```python
from build123d import *

# Parameters (mm, degrees)
SKETCH2_W             = 76.2
SKETCH2_H             = 6.15
BOSS_EXTRUDE1_DEPTH   = 28.575
BOSS_EXTRUDE1_2_DEPTH = 28.575
SKETCH2_3_W           = 76.2
SKETCH2_3_H           = 12.9
BOSS_EXTRUDE2_DEPTH   = 3.175
CUT_EXTRUDE2_DEPTH    = 90.858670283
SKETCH4_R             = 3.175
SKETCH4_R_2           = 2.38125
SKETCH4_R_3           = 1.5875
SKETCH4_R_4           = 0.79375
CUT_EXTRUDE3_DEPTH    = 90.858670283
SKETCH5_R             = 0.2
CUT_EXTRUDE4_DEPTH    = 90.858670283
CHAMFER1_SIZE         = 0.4
SKETCH6_W             = 76.2
SKETCH6_H             = 1
CUT_EXTRUDE5_DEPTH    = 0.79375


with BuildPart() as part:
    # Sketch2 → Boss-Extrude1 (new body)
    with BuildSketch(Plane(origin=(0, 0, 0), x_dir=(1, 0, 0), z_dir=(0, 1, 0))):
        with Locations((-38.1, 35.025)):
            Rectangle(SKETCH2_W, SKETCH2_H)
    extrude(amount=BOSS_EXTRUDE1_DEPTH)



with BuildPart() as body_2:
    # Sketch2 → Boss-Extrude1 2 (new body)
    with BuildSketch(Plane(origin=(0, 0, 0), x_dir=(1, 0, 0), z_dir=(0, 1, 0))):
        with Locations((-38.1, 3.075)):
            Rectangle(SKETCH2_W, SKETCH2_H)
    extrude(amount=BOSS_EXTRUDE1_2_DEPTH)


with BuildPart() as part_1:
    add(part.part)

    add(body_2.part)  # Boss-Extrude2 merges body 2
    # Sketch2_3 → Boss-Extrude2 (add)
    with BuildSketch(Plane(origin=(0, 0, 0), x_dir=(1, 0, 0), z_dir=(0, 1, 0))):
        with Locations((-38.1, 25.5)):
            Rectangle(SKETCH2_3_W, SKETCH2_3_H)
        with Locations((-38.1, 12.6)):
            Rectangle(SKETCH2_3_W, SKETCH2_3_H)
    extrude(amount=BOSS_EXTRUDE2_DEPTH)

    # Sketch3 → Cut-Extrude2 (cut, through all)
    with BuildSketch(Plane.XY):
        Polygon((-38.1, 9.525), (-38.1, 28.575), (-63.5, 28.575), (-50.8, 9.525), align=None)
        Polygon((-12.7, 28.575), (-38.1, 28.575), (-38.1, 9.525), (-25.4, 9.525), align=None)
    extrude(amount=-CUT_EXTRUDE2_DEPTH, mode=Mode.SUBTRACT)

    # Sketch4 → Cut-Extrude3 (cut, through all)
    with BuildSketch(Plane.XZ):
        with Locations(Location((-63.5, -19.05, 0), (0, 0, 270))):
            Circle(SKETCH4_R)
        with Locations(Location((-38.1, -19.05, 0), (0, 0, 270))):
            Circle(SKETCH4_R_2)
        with Locations(Location((-19.05, -19.05, 0), (0, 0, 270))):
            Circle(SKETCH4_R_3)
        with Locations(Location((-6.35, -19.05, 0), (0, 0, 270))):
            Circle(SKETCH4_R_4)
    extrude(amount=-CUT_EXTRUDE3_DEPTH, mode=Mode.SUBTRACT)

    # Sketch5 → Cut-Extrude4 (cut, through all)
    with BuildSketch(Plane(origin=(0, 0, 0), x_dir=(0, 0, -1), z_dir=(1, 0, 0))):
        with Locations((6.15, 3.175)):
            Circle(SKETCH5_R)
        with Locations((31.95, 3.175)):
            Circle(SKETCH5_R)
    extrude(amount=-CUT_EXTRUDE4_DEPTH, mode=Mode.SUBTRACT)

    # Chamfer1
    chamfer1_edges = [part_1.edges().sort_by_distance(p)[0] for p in [
        (-63.5, 0, -15.875),
        (-38.1, 0, -16.66875),
        (-19.05, 0, -17.4625),
        (-6.35, 0, -18.25625),
    ]]
    chamfer(chamfer1_edges, length=CHAMFER1_SIZE)

    # Sketch6 → Cut-Extrude5 (cut)
    with BuildSketch(Plane(origin=(0, 0, 0), x_dir=(-1, 0, 0), z_dir=(0, -1, 0))):
        with Locations((38.1, 19.05)):
            Rectangle(SKETCH6_W, SKETCH6_H)
    extrude(amount=-CUT_EXTRUDE5_DEPTH, mode=Mode.SUBTRACT)


solid = part_1.part
```
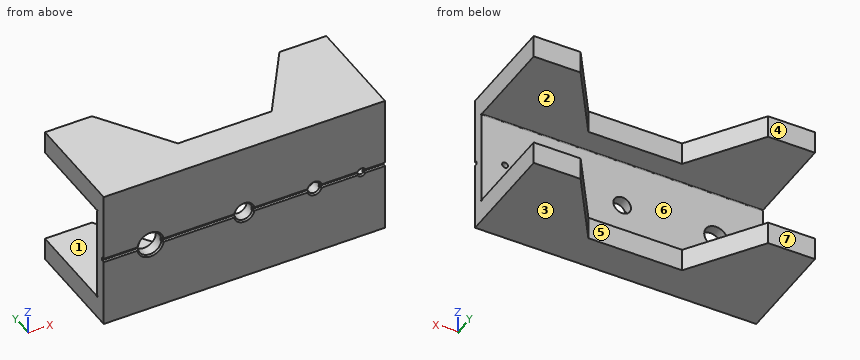
For this review, take the finished solid that the model builds, in its own axes (mm). Face numbers are marked on the shaded views. A direction names the side the tool comes from. Round coordinates to 2 decimals unless told otherwise and drop trailing zeros. Write each loop counter-clockwise with the first axis right and the second up, starting at its lowest first coordinate (ties: lowest second). Pieces come first, ordered by that corner, then holes. Notation, with made-up numbers: (-22, 38) - (-14, 38) arc R20 cw to (-14, 63) - close; hole circle Ø11 at (33, 21). An arc over 180 degrees is marked (long way). Put each result on its own line as item: value.
Q1. Wall thickness on probe 1 along X at (y, z) = (1.85, -19.05) (1 decimal); probe 2 along Z at (x, y) = (-13, 25.5): over which ranges is each line inside the solid? List them lowest first.
Solved:
probe 1: x = -76.2 to -66.7, -60.3 to -40.5, -35.7 to -20.6, -17.5 to -7.1, -5.6 to 0
probe 2: z = -38.1 to -31.95, -6.15 to 0
Q2. Machinability: for the marked faces 5, 6 and 7, which of the approach directions +Z, -Z, +X, -X, +Y, -Y give a long, thin tool a straight path to every point of the face, cutting with its end or side? Answer none if there is none.
Solved:
face 5: +Z, -Z, +Y
face 6: +X, -X, +Y
face 7: +Z, -Z, +X, -X, +Y
Q3. Mouldability with a two-part tool opening along Z and no side actions: class the marked faces 1, 2, 3 and 4 as released by +Z, released by -Z, zero draft, split by the parting line, or undercut.
Solved:
face 1: undercut
face 2: undercut
face 3: released by -Z
face 4: zero draft
Q4. We need section C-C (y = 14.5). Give the boundary of the cut face in (x, z), and give its area (3 significant figures).
Solved:
outline: (-76.2, -38.1) - (-54.12, -38.1) - (-54.12, -31.95) - (-76.2, -31.95) - close; (-76.2, -6.15) - (-54.12, -6.15) - (-54.12, 0) - (-76.2, 0) - close; (-22.08, -38.1) - (0, -38.1) - (0, -31.95) - (-22.08, -31.95) - close; (-22.08, -6.15) - (0, -6.15) - (0, 0) - (-22.08, 0) - close
area: 543 mm2
Q5. We need section D-D (z = -33). Give the boundary of the cut face in (x, y) (3 decimals), and give its area (3 significant figures).
Solved:
outline: (-76.2, 0) - (0, 0) - (0, 28.575) - (-12.7, 28.575) - (-25.4, 9.525) - (-50.8, 9.525) - (-63.5, 28.575) - (-76.2, 28.575) - close
area: 1,450 mm2
Q6. We need section A-A (x = -38.1). Give the boundary of the cut face in (y, z) (3 decimals).
Solved:
outline: (0, -38.1) - (9.525, -38.1) - (9.525, -31.95) - (3.375, -31.95) arc R0.2 cw (long way) to (3.175, -31.75) - (3.175, -21.431) - (0.4, -21.431) - (0, -21.831) - close; (0, -16.269) - (0.4, -16.669) - (3.175, -16.669) - (3.175, -6.35) arc R0.2 cw (long way) to (3.375, -6.15) - (9.525, -6.15) - (9.525, 0) - (0, 0) - close
Q7. Insertion check: pin 1 Ø0.8 at (x, z) = (-25, -19) entering from -Y; pin 2 Ø4 at (x, z) = (-19.05, -19.05) entering from +Y (3 decimals); pin 3 Ø1.8 at (x, z) = (-43, -4) entering from +Y (3 decimals). Each pin has a flat end and moves straight along its axis. Give the tip position at first contact, or say it passes through.
Solved:
pin 1: stops at y = 0.79
pin 2: stops at y = 3.175
pin 3: stops at y = 9.525
Q8. We need section B-B (y = 5.25). Give the boundary of the cut face in (x, z).
Solved:
outline: (-76.2, -38.1) - (0, -38.1) - (0, -31.95) - (-76.2, -31.95) - close; (-76.2, -6.15) - (0, -6.15) - (0, 0) - (-76.2, 0) - close
